Model file for the job. Use its own axes, mm. Coordinates: 2 decimals unless noted, no trailing zeros. Write each loop counter-clockwise with the first axis right and the second up, starting at its lowest first coordinate (ties: lowest second). Pieces come first, ordered by that corner, then holes.
Q1. Band-saw the part on A-A, the plane x = 21.5. Write the cut outline in (y, z).
Q2. Band-saw the part on C-C, the plane z = -21.5. Write the cut outline in (x, y), plus the area to 3 significant figures.
Q3. Pull direction Z, two halves, no side cores. Call faces 1 (the cylindrical face through (10.55, 0.99, -16.2)), 2 (the cylindrical face through (3.85, 1.01, -4.06)), 3 (the cylindrical face through (4.06, 1.01, -23.15)): released by +Z, released by -Z, zero draft, split by the parting line, or undercut.
Q4. Band-saw the part on B-B, the plane y = 0.65. State how many separate pieces and enclosed holes the cut face has, plus the area to 3 significant figures.
Q5. Drill centre lines: probe 1 along Z at (x, y) = (77.5, 0.75); probe 2 along Z at (x, y) = (21.5, 1.15); probe 3 along Z at (x, y) = (76, 0.25). Where is each one in solid material? Low to high.
Q6. Pin check, flat tips, straight feed: P1, Ø2, axis at x = 69.5, z = -13.5, coming from the +Y side; P2, Ø1, axis at y = 1.5, z = -23, coming from the +X side. Stop position of each tip, or through.
Q7. Band-saw the part on D-D, the plane x = 85.5. Write the cut outline in (y, z).
from build123d import *

# Parameters (mm, degrees)
SKETCH1_W                = 91
SKETCH1_H                = 27
EXTRUDE1_DEPTH           = 2
CUT_EXTRUDE1_START       = -2
CUT_EXTRUDE1_OUTLINE_R   = 4
CUT_EXTRUDE1_OUTLINE_R_2 = 1.85
CUT_EXTRUDE1_DEPTH       = 2
FILLET1_R                = 13.5
FILLET2_R                = 13.5
FILLET3_R                = 13.5
FILLET4_R                = 13.5


# Read off the part's stored shape, not the designer's step: Cut-Extrude1
with BuildPart() as part:
    # Sketch1 → Extrude1 (new body)
    with BuildSketch(Plane(origin=(0, 0, 0), x_dir=(1, 0, 0), z_dir=(0, 1, 0))):
        with Locations((45.5, 13.5)):
            Rectangle(SKETCH1_W, SKETCH1_H)
    extrude(amount=EXTRUDE1_DEPTH)

    # Cut-Extrude1 outline → Cut-Extrude1 (cut)
    with BuildSketch(Plane(origin=(0, 2, 0), x_dir=(1, 0, 0), z_dir=(0, 1, 0)).offset(CUT_EXTRUDE1_START)):
        with Locations((13.5, 13.5)):
            Circle(CUT_EXTRUDE1_OUTLINE_R)
        with Locations((21.5, 13.5)):
            Circle(CUT_EXTRUDE1_OUTLINE_R_2)
        with Locations((5.5, 13.5)):
            Circle(CUT_EXTRUDE1_OUTLINE_R_2)
        with Locations((13.5, 5.5)):
            Circle(CUT_EXTRUDE1_OUTLINE_R_2)
        with Locations((13.5, 21.5)):
            Circle(CUT_EXTRUDE1_OUTLINE_R_2)
        with Locations((77.5, 13.5)):
            Circle(CUT_EXTRUDE1_OUTLINE_R)
        with Locations((85.5, 13.5)):
            Circle(CUT_EXTRUDE1_OUTLINE_R_2)
        with Locations((69.5, 13.5)):
            Circle(CUT_EXTRUDE1_OUTLINE_R_2)
        with Locations((77.5, 5.5)):
            Circle(CUT_EXTRUDE1_OUTLINE_R_2)
        with Locations((77.5, 21.5)):
            Circle(CUT_EXTRUDE1_OUTLINE_R_2)
    extrude(amount=CUT_EXTRUDE1_DEPTH, mode=Mode.SUBTRACT)

    # Fillet1
    fillet1_edges = [part.edges().sort_by_distance(p)[0] for p in [
        (91, 1, 0),
    ]]
    fillet(fillet1_edges, radius=FILLET1_R)

    # Fillet2
    fillet2_edges = [part.edges().sort_by_distance(p)[0] for p in [
        (91, 1, -27),
    ]]
    fillet(fillet2_edges, radius=FILLET2_R - 0.0001)  # a hair under: the kernel refuses the full size

    # Fillet3
    fillet3_edges = [part.edges().sort_by_distance(p)[0] for p in [
        (0, 1, -27),
    ]]
    fillet(fillet3_edges, radius=FILLET3_R)

    # Fillet4
    fillet4_edges = [part.edges().sort_by_distance(p)[0] for p in [
        (0, 1, 0),
    ]]
    fillet(fillet4_edges, radius=FILLET4_R - 0.0001)  # a hair under: the kernel refuses the full size


solid = part.part
Answer sheet:
1. outline: (0, -27) - (2, -27) - (2, -15.35) - (0, -15.35) - close; (0, -11.65) - (2, -11.65) - (2, 0) - (0, 0) - close
2. outline: (2.63, 0) - (11.65, 0) - (11.65, 2) - (2.63, 2) - close; (15.35, 0) - (75.65, 0) - (75.65, 2) - (15.35, 2) - close; (79.35, 0) - (88.37, 0) - (88.37, 2) - (79.35, 2) - close
2. area: 157 mm2
3. face 1: undercut
3. face 2: released by +Z
3. face 3: released by -Z
4. separate pieces: 1
4. enclosed holes: 10
4. area: 2,110 mm2
5. probe 1: z = -27 to -23.35, -19.65 to -17.5, -9.5 to -7.35, -3.65 to 0
5. probe 2: z = -27 to -15.35, -11.65 to 0
5. probe 3: z = -27 to -22.58, -20.42 to -17.21, -9.79 to -6.58, -4.42 to 0
6. P1: passes through
6. P2: stops at x = 87.56
7. outline: (0, -24.37) - (2, -24.37) - (2, -15.35) - (0, -15.35) - close; (0, -11.65) - (2, -11.65) - (2, -2.63) - (0, -2.63) - close
